```python
from build123d import *

# Parameters (mm, degrees)
SKETCH1_W                  = 31.75
SKETCH1_H                  = 101.6
BASE_FLANGE1_DEPTH         = 2.54
CUT_EXTRUDE1_DEPTH         = 107.475697227
FILLET1_R                  = 2.54
FILLET2_R                  = 2.54
SKETCH7_R                  = 3.302
CUT_EXTRUDE2_DEPTH         = 2.54
SKETCHED_START             = 61.806879931
SKETCHED_BEND7_OUTLINE_W   = 2.54
SKETCHED_BEND7_OUTLINE_H   = 22.225
SKETCHED_BEND7_DEPTH       = 27.093120069
SKETCHED_START_2           = 59.736360831
SKETCHED_BEND7_2_DEPTH     = 2.0705191
SKETCHED_START_3           = 57.831360831
SKETCHED_BEND7_3_DEPTH     = 4.445
SKETCHED_START_4           = -33
SKETCHED_BEND7_4_DEPTH     = 23.475
SKETCHED_START_5           = -31.75
SKETCHED_BEND7_5_DEPTH     = 22.225
SKETCHED_START_6           = 90.216360831
SKETCHED_BEND8_OUTLINE_W   = 2.54
SKETCHED_BEND8_OUTLINE_H   = 31.75
SKETCHED_BEND8_DEPTH       = 11.383639169
SKETCHED_START_7           = 87.676360831
SKETCHED_BEND8_2_DEPTH     = 2.0705191
SKETCHED_START_8           = 89.948086031
SKETCHED_BEND8_3_OUTLINE_W = 2.54
SKETCHED_BEND8_3_OUTLINE_H = 6.985
SKETCHED_BEND8_3_DEPTH     = 0.2682748
SKETCHED_START_9           = 85.771360831
SKETCHED_BEND8_4_DEPTH     = 4.445
SKETCHED_BEND8_5_DEPTH     = 31.75


with BuildPart() as part:
    # Base-Flange1: sheet metal written as solids
    # Sketch1 → Base-Flange1 (new body)
    with BuildSketch(Plane(origin=(0, 0, 0), x_dir=(0, 0, -1), z_dir=(1, 0, 0))):
        with Locations((15.875, 50.8)):
            Rectangle(SKETCH1_W, SKETCH1_H)
    extrude(amount=-BASE_FLANGE1_DEPTH)

    # Sketch6 → Cut-Extrude1 (cut, through all)
    with BuildSketch(Plane(origin=(0, 0, 0), x_dir=(0, 0, -1), z_dir=(1, 0, 0))):
        with BuildLine():
            Line((31.75, 88.9), (12.065, 88.9))
            ThreePointArc((12.065, 88.9), (10.268948776, 88.156051224), (9.525, 86.36))
            Line((9.525, 86.36), (9.525, 57.15))
            Line((9.525, 57.15), (6.985, 57.15))
            Line((6.985, 57.15), (6.985, 91.44))
            Line((6.985, 91.44), (31.75, 91.44))
            Line((31.75, 91.44), (31.75, 88.9))
        make_face()
    extrude(amount=-CUT_EXTRUDE1_DEPTH, mode=Mode.SUBTRACT)

    # Fillet1
    fillet1_edges = [part.edges().sort_by_distance(p)[0] for p in [
        (-1.27, 88.9, -31.75),
    ]]
    fillet(fillet1_edges, radius=FILLET1_R)

    # Fillet2
    fillet2_edges = [part.edges().sort_by_distance(p)[0] for p in [
        (-1.27, 91.44, -31.75),
        (-1.27, 101.6, 0),
        (-1.27, 101.6, -31.75),
        (-1.27, 0, -31.75),
        (-1.27, 0, 0),
    ]]
    fillet(fillet2_edges, radius=FILLET2_R)

    # Sketch7 → Cut-Extrude2 (cut)
    with BuildSketch(Plane(origin=(0, 0, 0), x_dir=(0, 0, -1), z_dir=(1, 0, 0))):
        with Locations((6.35, 12.7)):
            Circle(SKETCH7_R)
        with Locations((25.4, 12.7)):
            Circle(SKETCH7_R)
    extrude(amount=-CUT_EXTRUDE2_DEPTH, mode=Mode.SUBTRACT)

    # Sketched Bend7: read off the stored shape, not the designer's step
    # Sketched Bend7 outline → Sketched Bend7 (cut)
    with BuildSketch(Plane(origin=(0, 0, 0), x_dir=(1, 0, 0), z_dir=(0, 1, 0)).offset(SKETCHED_START)):
        with Locations((-1.27, 20.6375)):
            Rectangle(SKETCHED_BEND7_OUTLINE_W, SKETCHED_BEND7_OUTLINE_H)
    extrude(amount=SKETCHED_BEND7_DEPTH, mode=Mode.SUBTRACT)

    # Sketched Bend7 2 outline → Sketched Bend7 2 (add)
    with BuildSketch(Plane(origin=(0, 0, 0), x_dir=(1, 0, 0), z_dir=(0, 1, 0)).offset(SKETCHED_START_2)):
        with BuildLine():
            Line((0, 9.525), (25.446360831, 9.525))
            ThreePointArc((25.446360831, 9.525), (27.242412055, 10.268948776), (27.986360831, 12.065))
            Line((27.986360831, 12.065), (27.986360831, 29.21))
            ThreePointArc((27.986360831, 29.21), (27.242412055, 31.006051224), (25.446360831, 31.75))
            Line((25.446360831, 31.75), (0, 31.75))
            Line((0, 31.75), (0, 9.525))
        make_face()
    extrude(amount=SKETCHED_BEND7_2_DEPTH)

    # Sketched Bend7 3 outline → Sketched Bend7 3 (add)
    with BuildSketch(Plane(origin=(0, 0, 0), x_dir=(1, 0, 0), z_dir=(0, 1, 0)).offset(SKETCHED_START_3)):
        with BuildLine():
            Line((0, 9.525), (25.446360831, 9.525))
            ThreePointArc((25.446360831, 9.525), (27.242412055, 10.268948776), (27.986360831, 12.065))
            Line((27.986360831, 12.065), (27.986360831, 29.21))
            ThreePointArc((27.986360831, 29.21), (27.242412055, 31.006051224), (25.446360831, 31.75))
            Line((25.446360831, 31.75), (0, 31.75))
            Line((0, 31.75), (0, 9.525))
        make_face()
    extrude(amount=SKETCHED_BEND7_3_DEPTH)

    # Sketched Bend7 4 outline → Sketched Bend7 4 (cut)
    with BuildSketch(Plane.XY.offset(SKETCHED_START_4)):
        with BuildLine():
            Line((27.986360831, 57.831360831), (27.986360831, 59.736360831))
            Line((27.986360831, 59.736360831), (1.905, 59.736360831))
            ThreePointArc((1.905, 59.736360831), (0.557961582, 59.178399249), (0, 57.831360831))
            Line((0, 57.831360831), (27.986360831, 57.831360831))
        make_face()
        with BuildLine():
            ThreePointArc((-2.54, 57.831360831), (-1.876266121, 60.168036145), (-0.083283905, 61.806879931))
            Line((-0.083283905, 61.806879931), (-2.54, 61.806879931))
            Line((-2.54, 61.806879931), (-2.54, 57.831360831))
        make_face()
        with BuildLine():
            ThreePointArc((0, 61.84745346), (0.928656498, 62.167808498), (1.905, 62.276360831))
            Line((1.905, 62.276360831), (0, 62.276360831))
            Line((0, 62.276360831), (0, 61.84745346))
        make_face()
    extrude(amount=SKETCHED_BEND7_4_DEPTH, mode=Mode.SUBTRACT)

    # Sketched Bend7 5 outline → Sketched Bend7 5 (add)
    with BuildSketch(Plane.XY.offset(SKETCHED_START_5)):
        with BuildLine():
            Line((0, 61.806879931), (0, 61.84745346))
            ThreePointArc((0, 61.84745346), (-0.041747658, 61.827383673), (-0.083283905, 61.806879931))
            Line((-0.083283905, 61.806879931), (0, 61.806879931))
        make_face()
    extrude(amount=SKETCHED_BEND7_5_DEPTH)

    # Sketched Bend8: read off the stored shape, not the designer's step
    # Sketched Bend8 outline → Sketched Bend8 (cut)
    with BuildSketch(Plane(origin=(0, 0, 0), x_dir=(1, 0, 0), z_dir=(0, 1, 0)).offset(SKETCHED_START_6)):
        with Locations((-1.27, 15.875)):
            Rectangle(SKETCHED_BEND8_OUTLINE_W, SKETCHED_BEND8_OUTLINE_H)
    extrude(amount=SKETCHED_BEND8_DEPTH, mode=Mode.SUBTRACT)

    # Sketched Bend8 2 outline → Sketched Bend8 2 (add)
    with BuildSketch(Plane(origin=(0, 0, 0), x_dir=(1, 0, 0), z_dir=(0, 1, 0)).offset(SKETCHED_START_7)):
        with BuildLine():
            Line((0, 6.985), (0, 0))
            Line((0, 0), (10.206360831, 0))
            ThreePointArc((10.206360831, 0), (12.002412055, 0.743948776), (12.746360831, 2.54))
            Line((12.746360831, 2.54), (12.746360831, 29.21))
            ThreePointArc((12.746360831, 29.21), (12.002412055, 31.006051224), (10.206360831, 31.75))
            Line((10.206360831, 31.75), (5.126360831, 31.75))
            ThreePointArc((5.126360831, 31.75), (3.330309607, 31.006051224), (2.586360831, 29.21))
            Line((2.586360831, 29.21), (2.586360831, 6.985))
            Line((2.586360831, 6.985), (0, 6.985))
        make_face()
    extrude(amount=SKETCHED_BEND8_2_DEPTH)

    # Sketched Bend8 3 outline → Sketched Bend8 3 (cut)
    with BuildSketch(Plane(origin=(0, 0, 0), x_dir=(1, 0, 0), z_dir=(0, 1, 0)).offset(SKETCHED_START_8)):
        with Locations((-1.27, 3.4925)):
            Rectangle(SKETCHED_BEND8_3_OUTLINE_W, SKETCHED_BEND8_3_OUTLINE_H)
    extrude(amount=SKETCHED_BEND8_3_DEPTH, mode=Mode.SUBTRACT)

    # Sketched Bend8 4 outline → Sketched Bend8 4 (add)
    with BuildSketch(Plane(origin=(0, 0, 0), x_dir=(1, 0, 0), z_dir=(0, 1, 0)).offset(SKETCHED_START_9)):
        with BuildLine():
            Line((0, 0), (10.206360831, 0))
            ThreePointArc((10.206360831, 0), (12.002412055, 0.743948776), (12.746360831, 2.54))
            Line((12.746360831, 2.54), (12.746360831, 29.21))
            ThreePointArc((12.746360831, 29.21), (12.002412055, 31.006051224), (10.206360831, 31.75))
            Line((10.206360831, 31.75), (5.126360831, 31.75))
            ThreePointArc((5.126360831, 31.75), (3.330309607, 31.006051224), (2.586360831, 29.21))
            Line((2.586360831, 29.21), (2.586360831, 6.985))
            Line((2.586360831, 6.985), (0, 6.985))
            Line((0, 6.985), (0, 0))
        make_face()
    extrude(amount=SKETCHED_BEND8_4_DEPTH)

    # Sketched Bend8 5 outline → Sketched Bend8 5 (cut)
    with BuildSketch(Plane.XY.offset(SKETCHED_START_5)):
        with BuildLine():
            Line((-2.54, 89.948086031), (-2.54, 85.771360831))
            ThreePointArc((-2.54, 85.771360831), (-1.238089643, 88.914450473), (1.905, 90.216360831))
            Line((1.905, 90.216360831), (0, 90.216360831))
            Line((0, 90.216360831), (0, 89.948086031))
            Line((0, 89.948086031), (-2.54, 89.948086031))
        make_face()
        with BuildLine():
            Line((0, 85.771360831), (12.746360831, 85.771360831))
            Line((12.746360831, 85.771360831), (12.746360831, 87.676360831))
            Line((12.746360831, 87.676360831), (1.905, 87.676360831))
            ThreePointArc((1.905, 87.676360831), (0.557961582, 87.118399249), (0, 85.771360831))
        make_face()
    extrude(amount=SKETCHED_BEND8_5_DEPTH, mode=Mode.SUBTRACT)


solid = part.part
```
Work out the finished part from the listing and answer in its coordinate system (mm). A direction names the side the tool comes from. Give positions to 0.01 mm unless a question says otherwise; leave off trailing zeros. Write each loop counter-clockwise with the first axis right and the second up, starting at its lowest first coordinate (ties: lowest second). Pieces come first, ordered by that corner, then holes.
(1) Which of the six approach directions +Z, -Z, +X, -X, +Y, -Y give full straight-line access (tool end or side, diameter ignored) to faces 1 (the cylindrical face through (12.02, 88.93, -30.99)), 2 (the cylindrical face through (-1.894, 60.139, -20.793)), 3 (the flat face through (15, 59.736, -21)), 4 (the cylindrical face through (-1.288, 0.724, -0.764)), 5 (the flat face through (-1, 39, -31.75))?
Final values:
face 1: -Z, +X, +Y
face 2: -Z, -X, +Y
face 3: +Z, -Z, +X, -Y
face 4: +Z, +X, -X, -Y
face 5: -Z, +X, -X, +Y, -Y
(2) The part is cut by section A-A on y = 12.7. Write down the section's boundary in (x, z), plus the area to 3 significant figures.
Final values:
outline: (-2.54, -31.75) - (0, -31.75) - (0, -28.7) - (-2.54, -28.7) - close; (-2.54, -22.1) - (0, -22.1) - (0, -9.65) - (-2.54, -9.65) - close; (-2.54, -3.05) - (0, -3.05) - (0, 0) - (-2.54, 0) - close
area: 47.1 mm2
(3) The part is cut by section C-C on x = 6.5. Write down the section's boundary in (y, z) (3 decimals).
Final values:
outline: (59.736, -31.75) - (62.276, -31.75) - (62.276, -9.525) - (59.736, -9.525) - close; (87.676, -31.75) - (90.216, -31.75) - (90.216, 0) - (87.676, 0) - close
(4) The mould has two halves that part along Y. Classify faces 6 (the flat face through (12.746, 89, -16)), 7 (the flat face through (7, 87.676, -16)), 8 (the flat face through (-1, 0, -16)): pulls with the +Y half, pulls with the -Y half, needs draft (parallel to the pull), parting line crosses it, or undercut.
Final values:
face 6: needs draft
face 7: undercut
face 8: pulls with the -Y half
(5) Flat-ended cylindrical pins translate along their axes: pin 1 Ø4 at (y, z) = (12.7, -25.4) entering from -X; pin 2 Ø1.3 at (x, z) = (-0.5, -8.5) entering from +Y; pin 3 Ø11 at (x, z) = (18.5, -21.5) entering from -Y; pin 4 Ø3 at (y, z) = (89, -20) entering from -X. Find the tip coordinate at first contact, or state that the pin passes through.
Final values:
pin 1: passes through
pin 2: stops at y = 57.15
pin 3: stops at y = 59.74
pin 4: stops at x = 2.59
(6) The part is cut by section D-D on y = 49. Write down the section's boundary in (x, z), plus the area to 3 significant figures.
Final values:
outline: (-2.54, -31.75) - (0, -31.75) - (0, 0) - (-2.54, 0) - close
area: 80.6 mm2
(7) The part is cut by section B-B on z = -25.4. Write down the section's boundary in (x, y) (3 decimals).
Final values:
outline: (-2.54, 0) - (0, 0) - (0, 9.398) - (-2.54, 9.398) - close; (-2.54, 16.002) - (0, 16.002) - (0, 57.831) arc R1.905 cw to (1.905, 59.736) - (27.986, 59.736) - (27.986, 62.276) - (1.905, 62.276) arc R4.445 ccw to (0, 61.847) arc R4.445 ccw to (-0.083, 61.807) arc R4.445 ccw to (-2.54, 57.831) - close; (2.586, 87.676) - (12.746, 87.676) - (12.746, 90.216) - (2.586, 90.216) - close
(8) Straight lines are drawn through the part: line 1 (Z direction, x = -1, y = 12); line 2 (X direction, y = 42, z = -30); line 3 (Y direction, x = 6, z = -5.5). For each, find the intervals that lie inside material, in ascending order.
Final values:
line 1: z = -31.75 to -28.63, -22.17 to -9.58, -3.12 to 0
line 2: x = -2.54 to 0
line 3: y = 87.68 to 90.22
